Check sheet for the modelled part. Datum: model origin and axes. Units: mm. A direction names the side the tool comes from. Round coordinates to 2 decimals unless told otherwise and drop trailing zeros. Order: outer loops, then holes, each group sorted by start corner. A loop starts at its lowest first (then second) coordinate and runs counter-clockwise, first axis right, second up.
(1) Depth check by flat-ended pin: pin 1 (12 mm diameter, centred on y = 36.5, z = -9.5, fed in from -X); pin 2 (8 mm diameter, centred on y = 6.5, z = 7, fed in from +X); pin 3 (5 mm diameter, centred on y = 39.5, z = 5.5, fed in from -X); pin 4 (6 mm diameter, centred on x = 0, z = 0, fed in from +Y). Enter the tip coordinate at first touch or a pass-through.
(2) Thickness scan on probe 1 along Z at (x, y) = (0, 20); probe 2 along Z at (x, y) = (0, 42.5). Record the ranges inside material, lowest first.
(3) Tool access check on faces 4 (the flat face through (3, 45.5, 3)), 5 (the cylindrical face through (-8.05, 27.93, 6.18)), 6 (the cylindrical face through (5.589, 20.964, 2.317)). Record the directions out of +Z, -Z, +X, -X, +Y, -Y that give a thin tool (end or side, any length) a straight path to the whole face; none if there is none.
(4) Mould release check, pull along Z, two halves, no side actions. Record for faces 1 (the flat face through (3, 41.349, -3)), 2 (the conical face through (6.19, 45.42, 1.95)), 3 (the flat face through (3, 5.2, -10)): released by +Z, released by -Z, zero draft, split by the parting line, or undercut.
(5) Sectioned sample at A-A, the plane x = 0. Enter the section's corners in (y, z), and give its area (3 significant figures).
(6) Sectioned sample at C-C, the plane y = 28.5. Enter the section's corners in (x, z), and give its area (3 significant figures).
(7) Sectioned sample at B-B, the plane z = 0. Enter the section's corners in (x, y).
Autodesk Inventor part; units mm, degrees
ref_plane "XZ Plane" through (0, 0, 0) normal (0, 1, 0) x (-1, 0, 0)
sketch "Sketch1" plane through (0, 0, 0) normal (0, 0, 1) x (1, 0, 0)
  line L0 (6.05, 0) -> (6.05, 41.3489)
  line L1 (6.05, 0) -> (10.15, 0)
  line L2 (10.15, 0) -> (10.15, 5.2)
  line L3 (10.15, 5.2) -> (11.8, 5.2)
  line L4 (11.8, 5.2) -> (11.8, 11.2)
  line L5 (11.8, 11.2) -> (10.15, 11.2)
  line L6 (0, -9.1) -> (0, 54.6) construction
  line L7 (10.15, 11.2) -> (10.15, 44.2)
  line L8 (6.25, 45.5) -> (10.15, 44.2)
  line L9 (6.25, 45.5) -> (3.75, 45.5)
  line L10 (3.75, 45.5) -> (3.75, 41.3489)
  line L11 (3.75, 41.3489) -> (6.05, 41.3489)
  point P0 (0, 0)
  dimension "d0" = 10.15
  dimension "d1" = 4.1
  dimension "d2" = 11.2
  dimension "d3" = 11.8
  dimension "d5" = 6.05
  dimension "d9" = 44.2
  dimension "d11" = 45.5
  dimension "d13" = 6
  dimension "d14" = 3.75
  dimension "d15" = 4.1511
  dimension "d16" = 6.25
revolve "Revolution1" add sketch "Sketch1" angle 360 about axis through (0, -10, 0) along (0, 1, 0)
properties part number "Objective-Lens"
Derived:
1. pin 1: stops at x = -9.53
1. pin 2: stops at x = 11.41
1. pin 3: stops at x = -9.7
1. pin 4: passes through
2. probe 1: z = -10.15 to -6.05, 6.05 to 10.15
2. probe 2: z = -10.15 to -3.75, 3.75 to 10.15
3. face 4: +Z, -Z, +X, -X, +Y
3. face 5: +Y
3. face 6: -Y
4. face 1: undercut
4. face 2: split by the parting line
4. face 3: zero draft
5. outline: (0, -10.15) - (5.2, -10.15) - (5.2, -11.8) - (11.2, -11.8) - (11.2, -10.15) - (44.2, -10.15) - (45.5, -6.25) - (45.5, -3.75) - (41.35, -3.75) - (41.35, -6.05) - (0, -6.05) - close; (0, 6.05) - (41.35, 6.05) - (41.35, 3.75) - (45.5, 3.75) - (45.5, 6.25) - (44.2, 10.15) - (11.2, 10.15) - (11.2, 11.8) - (5.2, 11.8) - (5.2, 10.15) - (0, 10.15) - close
5. area: 407 mm2
6. outline: circle Ø20.3 at (0, 0); hole circle Ø12.1 at (0, 0)
6. area: 209 mm2
7. outline: (-11.8, 5.2) - (-10.15, 5.2) - (-10.15, 0) - (-6.05, 0) - (-6.05, 41.35) - (-3.75, 41.35) - (-3.75, 45.5) - (-6.25, 45.5) - (-10.15, 44.2) - (-10.15, 11.2) - (-11.8, 11.2) - close; (3.75, 41.35) - (6.05, 41.35) - (6.05, 0) - (10.15, 0) - (10.15, 5.2) - (11.8, 5.2) - (11.8, 11.2) - (10.15, 11.2) - (10.15, 44.2) - (6.25, 45.5) - (3.75, 45.5) - close
